Design review of the part built by this model. Coordinates are the model's own, in mm. Give positions to 0.01 mm unless a question says otherwise; leave off trailing zeros. Write each loop counter-clockwise with the first axis right and the second up, starting at its lowest first coordinate (ties: lowest second). Pieces come first, ordered by that corner, then holes. Notation, with made-up numbers: (-19.5, 43.25) -> (39.5, 43.25) arc R13 ccw to (39.5, 61.25) -> close; hole circle Ø9 at (1.25, 1). An arc over 180 degrees is marked (long way). Put each result on its own line as item: value. Start each with the question number.
from build123d import *

# Parameters (mm, degrees)
SKETCH1_R           = 1.5
SKETCH1_W           = 0.5
SKETCH1_H           = 0.5
SKETCH1_W_2         = 0.65
SKETCH1_H_2         = 0.63
BOSS_EXTRUDE1_DEPTH = 2


with BuildPart() as part:
    # Sketch1 → Boss-Extrude1 (new body)
    with BuildSketch(Plane(origin=(0, 0, 0), x_dir=(1, 0, 0), z_dir=(0, 1, 0))):
        Polygon((-19, 5), (-19, -6), (-16, -9), (16, -9), (19, -6), (19, 5), (16, 8), (-16, 8), align=None)
        with Locations((-7, -3)):
            Circle(SKETCH1_R, mode=Mode.SUBTRACT)
        with Locations((7, -3)):
            Circle(SKETCH1_R, mode=Mode.SUBTRACT)
        with Locations((0, 5)):
            Circle(SKETCH1_R, mode=Mode.SUBTRACT)
        with Locations((-16.27, 2.75)):
            Rectangle(SKETCH1_W, SKETCH1_H, mode=Mode.SUBTRACT)
        with Locations((-16.27, -2.75)):
            Rectangle(SKETCH1_W, SKETCH1_H, mode=Mode.SUBTRACT)
        with Locations((-13.73, -2.75)):
            Rectangle(SKETCH1_W, SKETCH1_H, mode=Mode.SUBTRACT)
        with Locations((-13.73, 2.75)):
            Rectangle(SKETCH1_W, SKETCH1_H, mode=Mode.SUBTRACT)
        with Locations((13.73, 2.75)):
            Rectangle(SKETCH1_W, SKETCH1_H, mode=Mode.SUBTRACT)
        with Locations((13.73, -2.75)):
            Rectangle(SKETCH1_W, SKETCH1_H, mode=Mode.SUBTRACT)
        with Locations((16.27, -2.75)):
            Rectangle(SKETCH1_W, SKETCH1_H, mode=Mode.SUBTRACT)
        with Locations((16.27, 2.75)):
            Rectangle(SKETCH1_W, SKETCH1_H, mode=Mode.SUBTRACT)
        with Locations((-3.81, -6.934)):
            Rectangle(SKETCH1_W_2, SKETCH1_H_2, mode=Mode.SUBTRACT)
        with Locations((-1.27, -6.934)):
            Rectangle(SKETCH1_W_2, SKETCH1_H_2, mode=Mode.SUBTRACT)
        with Locations((1.27, -6.934)):
            Rectangle(SKETCH1_W_2, SKETCH1_H_2, mode=Mode.SUBTRACT)
        with Locations((3.81, -6.934)):
            Rectangle(SKETCH1_W_2, SKETCH1_H_2, mode=Mode.SUBTRACT)
    extrude(amount=BOSS_EXTRUDE1_DEPTH)


solid = part.part
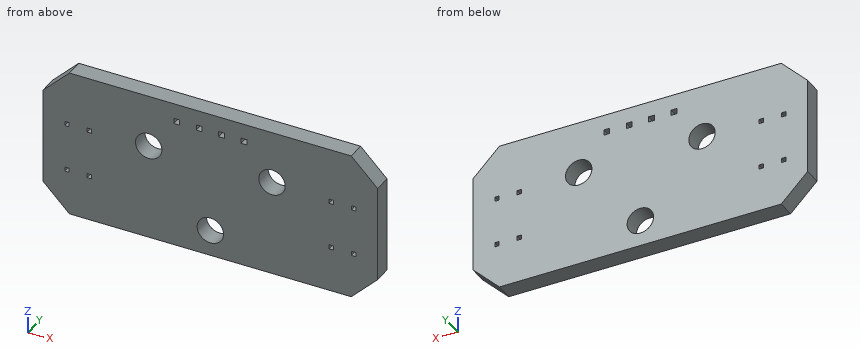
Q1. Take a section at C-C on y = 1.7. State how many separate pieces and enclosed holes the cut face has, then the cut area to 3 significant figures.
Q2. Take a section at B-B on z = 8.25. Give the boundary of the cut face in (x, y), then the cut area to 3 significant figures.
Q3. To check wall thickness, follow probe 1 along Z at (x, y) = (-7, 0.65); probe 2 along Z at (x, y) = (0, 1.2); probe 3 along X at (y, z) = (0.25, 7) (3 decimals). State the ranges of each line that lie inside material, in increasing order. Write a range as from..to.
Q4. Take a section at A-A on x = 7. Give the boundary of the cut face in (y, z), then the cut area to 3 significant figures.
Q5. For pin 1 (3.5 mm diameter, centred on x = 7, z = 3, fed in from -Y); pin 2 (0.5 mm diameter, centred on y = 1, z = 7, fed in from -X), all flat-tipped, find the tip position at first contact; note any pin that passes through.
Result:
1. separate pieces: 1
1. enclosed holes: 15
1. area: 603 mm^2
2. outline: (-16.75, 0) -> (16.75, 0) -> (16.75, 2) -> (-16.75, 2) -> close
2. area: 67.0 mm^2
3. probe 1: z = -8..1.5, 4.5..9
3. probe 2: z = -8..-6.5, -3.5..9
3. probe 3: x = -18..-4.135, -3.485..-1.595, -0.945..0.945, 1.595..3.485, 4.135..18
4. outline: (0, -8) -> (2, -8) -> (2, 1.5) -> (0, 1.5) -> close; (0, 4.5) -> (2, 4.5) -> (2, 9) -> (0, 9) -> close
4. area: 28.0 mm^2
5. pin 1: stops at y = 0
5. pin 2: stops at x = -18.25
